Can you work these out from the model? Positions are in its coordinate system, mm. A direction names the side the tool comes from. Round coordinates to 2 decimals unless told otherwise and drop trailing zeros. Order: outer loops, then holes, each group sorted by start corner. A loop starts at its lowest first (then second) coordinate and runs counter-clockwise, first axis right, second up. Notation, with made-up numbers: (-11, -22.75) -> (19, -22.75) arc R26 ccw to (19, 4.25) -> close; hole circle Ø2 at (23, -21.75). An arc over 180 degrees is marked (long way). One line per item, written item: value.
```python
from build123d import *

# Parameters (mm, degrees)
SKETCH_W        = 50
SKETCH_H        = 50
SKETCH_W_2      = 46
SKETCH_H_2      = 46
PAD_DEPTH       = 20
SKETCH001_W     = 50
SKETCH001_H     = 50
PAD001_DEPTH    = 4
SKETCH002_W     = 27
SKETCH002_H     = 18
POCKET_DEPTH    = 5
CHAMFER_SIZE    = 2
CHAMFER001_SIZE = 2
PAD002_DEPTH    = 15
CHAMFER002_SIZE = 2


with BuildPart() as part:
    # Sketch → Pad (new body)
    with BuildSketch(Plane.XY):
        Rectangle(SKETCH_W, SKETCH_H)
        Rectangle(SKETCH_W_2, SKETCH_H_2, mode=Mode.SUBTRACT)
    extrude(amount=PAD_DEPTH)

    # Sketch001 (on Face10 of Pad) → Pad001 (join)
    with BuildSketch(Plane.XY.offset(20)):
        Rectangle(SKETCH001_W, SKETCH001_H)
    extrude(amount=PAD001_DEPTH)

    # Sketch002 (on Face6 of Pad001) → Pocket (cut)
    with BuildSketch(Plane.XZ.offset(25)):
        with Locations((0, 9)):
            Rectangle(SKETCH002_W, SKETCH002_H)
    extrude(amount=-POCKET_DEPTH, mode=Mode.SUBTRACT)

    # Chamfer
    chamfer_edges = [part.edges().sort_by_distance(p)[0] for p in [
        (-25, -25, 22),
        (-25, -25, 10),
        (25, -25, 10),
        (25, -25, 22),
        (25, 25, 10),
        (25, 25, 22),
        (-25, 25, 10),
        (-25, 25, 22),
        (-23, 23, 10),
        (23, -23, 10),
        (23, 23, 10),
        (-23, -23, 10),
    ]]
    chamfer(chamfer_edges, length=CHAMFER_SIZE)

    # Chamfer001
    chamfer001_edges = [part.edges().sort_by_distance(p)[0] for p in [
        (24, -24, 24),
        (-24, -24, 24),
        (24, 24, 24),
        (-24, 24, 24),
    ]]
    chamfer(chamfer001_edges, length=CHAMFER001_SIZE)

    # Sketch003 (on Face19 of Chamfer001) → Pad002 (join)
    with BuildSketch(Plane.XZ.offset(25)):
        Polygon((-13.5, 18), (-13.5, 0), (-15.5, 0), (-15.5, 20), (15.5, 20), (15.5, 0), (13.5, 0), (13.5, 18), align=None)
    extrude(amount=PAD002_DEPTH)

    # Chamfer002
    chamfer002_edges = [part.edges().sort_by_distance(p)[0] for p in [
        (13.5, -32.5, 18),
        (-13.5, -32.5, 18),
        (15.5, -32.5, 20),
        (-15.5, -32.5, 20),
    ]]
    chamfer(chamfer002_edges, length=CHAMFER002_SIZE)


solid = part.part
```
Q1. I want a section at A-A on y = -29. List the corners of the cut face in (x, z) for me, plus the area to 3 significant figures.
Answers below:
outline: (-15.5, 0) -> (-13.5, 0) -> (-13.5, 16) -> (-11.5, 18) -> (11.5, 18) -> (13.5, 16) -> (13.5, 0) -> (15.5, 0) -> (15.5, 18) -> (13.5, 20) -> (-13.5, 20) -> (-15.5, 18) -> close
area: 134 mm^2
Q2. I want a section at B-B on x = -0.5. List the corners of the cut face in (y, z) for me, plus the area to 3 significant figures.
Answers below:
outline: (-40, 18) -> (-23, 18) -> (-23, 20) -> (23, 20) -> (23, 0) -> (25, 0) -> (25, 24) -> (-25, 24) -> (-25, 20) -> (-40, 20) -> close
area: 274 mm^2
Q3. I want a section at D-D on y = -0.5. List the corners of the cut face in (x, z) for me, plus the area to 3 significant figures.
Answers below:
outline: (-25, 0) -> (-23, 0) -> (-23, 20) -> (23, 20) -> (23, 0) -> (25, 0) -> (25, 24) -> (-25, 24) -> close
area: 280 mm^2
Q4. Will these pins go through, and if not, where does the flat tip stop? pin 1 Ø7.5 at (y, z) = (-30, 13) entering from -X; pin 2 Ø4.5 at (x, y) = (3, -30) entering from +Z; pin 3 Ø5 at (x, y) = (-15, -12.5) entering from -Z.
Answers below:
pin 1: x = -15.5
pin 2: z = 20
pin 3: z = 20
Q5. I want a section at C-C on z = 3.75. List the corners of the cut face in (x, y) for me, plus the area to 3 significant figures.
Answers below:
outline: (-25, -23) -> (-23, -25) -> (-15.5, -25) -> (-15.5, -40) -> (-13.5, -40) -> (-13.5, -23) -> (-21, -23) -> (-23, -21) -> (-23, 21) -> (-21, 23) -> (21, 23) -> (23, 21) -> (23, -21) -> (21, -23) -> (13.5, -23) -> (13.5, -40) -> (15.5, -40) -> (15.5, -25) -> (23, -25) -> (25, -23) -> (25, 23) -> (23, 25) -> (-23, 25) -> (-25, 23) -> close
area: 390 mm^2
Q6. We'd pull the mould along Y, two halves only. Please class faces 1 (the face through (0, -31, 18)), 2 (the face through (22, -22, 10)), 3 (the face through (-24, 24, 11)): released by +Y, released by -Y, zero draft, split by the parting line, or undercut.
Answers below:
face 1: zero draft
face 2: undercut
face 3: released by +Y
Q7. Please list where these lines run through material, in increasing order: line 1 along Y through (x, z) = (16, 15.25); line 2 along Y through (x, z) = (-9.5, 7.25).
Answers below:
line 1: -25 to -23, 23 to 25
line 2: 23 to 25
Q8. On a 3-axis mill with a long thin cutter (end or side, diameter ignored), from which of +Z, -Z, +X, -X, +Y, -Y can I reach the whole of each face in a straight line? I mean faces 4 (the face through (-5, -25, 22)), 5 (the face through (-13.5, -31, 8)), 6 (the face through (-14.5, -32.4, 19)). Say none if no direction works.
Answers below:
face 4: +Z, -Y
face 5: -Z, -Y
face 6: +Z, -X, -Y
